```python
from build123d import *

# Parameters (mm, degrees)
F3_DEPTH = 32
F7_W     = 30
F7_H     = 8
F8_DEPTH = 4
F5_R     = 2.7
F9_DEPTH = 25


with BuildPart() as f1:
    # F0 (on Front) → F1 (revolve)
    with BuildSketch(Plane.XZ):
        Polygon((29.3, 16), (10.7, 16), (10.7, 13.35), (0, 13.35), (0, 0), (205, 0), (205, 12.5), (188.3, 12.5), (188.3, 12), (185.3, 12), (185.3, 14), (173.3, 14), (173.3, 13), (170.3, 13), (170.3, 14), (121.6, 14), (121.6, 13.3), (118.6, 13.3), (118.6, 16), (32.3, 16), (32.3, 15), (29.3, 15), align=None)
    revolve(axis=Axis((102.5, 0, 0), (-1, 0, 0)))

    # F2 (on face) → F3 (join)
    with BuildSketch(Plane(origin=(0, 0, 0), x_dir=(0, -1, 0), z_dir=(-1, 0, 0))):
        with BuildLine():
            ThreePointArc((-8.528071, 10.271052), (-6.675, 11.561439), (-4.630957, 12.521052))
            Line((-4.630957, 12.521052), (-5.630957, 14.253103))
            Line((-5.630957, 14.253103), (-9.146501, 16.842204))
            Line((-9.146501, 16.842204), (-10.012526, 16.342204))
            Line((-10.012526, 16.342204), (-9.528071, 12.003103))
            Line((-9.528071, 12.003103), (-8.528071, 10.271052))
        make_face()
        with BuildLine():
            Line((-2.25, 15.159027), (-2.25, 13.159027))
            ThreePointArc((-2.25, 13.159027), (0, 13.35), (2.25, 13.159027))
            Line((2.25, 13.159027), (2.25, 15.159027))
            Line((2.25, 15.159027), (0.5, 19.159027))
            Line((0.5, 19.159027), (-0.5, 19.159027))
            Line((-0.5, 19.159027), (-2.25, 15.159027))
        make_face()
        with BuildLine():
            Line((5.630957, 14.253103), (4.630957, 12.521052))
            ThreePointArc((4.630957, 12.521052), (6.675, 11.561439), (8.528071, 10.271052))
            Line((8.528071, 10.271052), (9.528071, 12.003103))
            Line((9.528071, 12.003103), (10.012526, 16.342204))
            Line((10.012526, 16.342204), (9.146501, 16.842204))
            Line((9.146501, 16.842204), (5.630957, 14.253103))
        make_face()
        with BuildLine():
            Line((12.003103, 9.528071), (10.271052, 8.528071))
            ThreePointArc((10.271052, 8.528071), (11.561439, 6.675), (12.521052, 4.630957))
            Line((12.521052, 4.630957), (14.253103, 5.630957))
            Line((14.253103, 5.630957), (16.842204, 9.146501))
            Line((16.842204, 9.146501), (16.342204, 10.012526))
            Line((16.342204, 10.012526), (12.003103, 9.528071))
        make_face()
        with BuildLine():
            Line((15.159027, 2.25), (13.159027, 2.25))
            ThreePointArc((13.159027, 2.25), (13.302171, 1.129045), (13.35, 0))
            ThreePointArc((13.35, 0), (13.302171, -1.129045), (13.159027, -2.25))
            Line((13.159027, -2.25), (15.159027, -2.25))
            Line((15.159027, -2.25), (19.159027, -0.5))
            Line((19.159027, -0.5), (19.159027, 0.5))
            Line((19.159027, 0.5), (15.159027, 2.25))
        make_face()
        with BuildLine():
            Line((14.253103, -5.630957), (12.521052, -4.630957))
            ThreePointArc((12.521052, -4.630957), (11.561439, -6.675), (10.271052, -8.528071))
            Line((10.271052, -8.528071), (12.003103, -9.528071))
            Line((12.003103, -9.528071), (16.342204, -10.012526))
            Line((16.342204, -10.012526), (16.842204, -9.146501))
            Line((16.842204, -9.146501), (14.253103, -5.630957))
        make_face()
        with BuildLine():
            Line((9.528071, -12.003103), (8.528071, -10.271052))
            ThreePointArc((8.528071, -10.271052), (6.675, -11.561439), (4.630957, -12.521052))
            Line((4.630957, -12.521052), (5.630957, -14.253103))
            Line((5.630957, -14.253103), (9.146501, -16.842204))
            Line((9.146501, -16.842204), (10.012526, -16.342204))
            Line((10.012526, -16.342204), (9.528071, -12.003103))
        make_face()
        with BuildLine():
            ThreePointArc((2.25, -13.159027), (0, -13.35), (-2.25, -13.159027))
            Line((-2.25, -13.159027), (-2.25, -15.159027))
            Line((-2.25, -15.159027), (-0.5, -19.159027))
            Line((-0.5, -19.159027), (0.5, -19.159027))
            Line((0.5, -19.159027), (2.25, -15.159027))
            Line((2.25, -15.159027), (2.25, -13.159027))
        make_face()
        with BuildLine():
            ThreePointArc((-4.630957, -12.521052), (-6.675, -11.561439), (-8.528071, -10.271052))
            Line((-8.528071, -10.271052), (-9.528071, -12.003103))
            Line((-9.528071, -12.003103), (-10.012526, -16.342204))
            Line((-10.012526, -16.342204), (-9.146501, -16.842204))
            Line((-9.146501, -16.842204), (-5.630957, -14.253103))
            Line((-5.630957, -14.253103), (-4.630957, -12.521052))
        make_face()
        with BuildLine():
            ThreePointArc((-10.271052, -8.528071), (-11.561439, -6.675), (-12.521052, -4.630957))
            Line((-12.521052, -4.630957), (-14.253103, -5.630957))
            Line((-14.253103, -5.630957), (-16.842204, -9.146501))
            Line((-16.842204, -9.146501), (-16.342204, -10.012526))
            Line((-16.342204, -10.012526), (-12.003103, -9.528071))
            Line((-12.003103, -9.528071), (-10.271052, -8.528071))
        make_face()
        with BuildLine():
            ThreePointArc((-13.159027, -2.25), (-13.35, 0), (-13.159027, 2.25))
            Line((-13.159027, 2.25), (-15.159027, 2.25))
            Line((-15.159027, 2.25), (-19.159027, 0.5))
            Line((-19.159027, 0.5), (-19.159027, -0.5))
            Line((-19.159027, -0.5), (-15.159027, -2.25))
            Line((-15.159027, -2.25), (-13.159027, -2.25))
        make_face()
        with BuildLine():
            ThreePointArc((-12.521052, 4.630957), (-11.561439, 6.675), (-10.271052, 8.528071))
            Line((-10.271052, 8.528071), (-12.003103, 9.528071))
            Line((-12.003103, 9.528071), (-16.342204, 10.012526))
            Line((-16.342204, 10.012526), (-16.842204, 9.146501))
            Line((-16.842204, 9.146501), (-14.253103, 5.630957))
            Line((-14.253103, 5.630957), (-12.521052, 4.630957))
        make_face()
        with BuildLine():
            ThreePointArc((2.25, 13.159027), (0, 13.35), (-2.25, 13.159027))
            ThreePointArc((-2.25, 13.159027), (-3.455234, 12.89511), (-4.630957, 12.521052))
            ThreePointArc((-4.630957, 12.521052), (-6.675, 11.561439), (-8.528071, 10.271052))
            ThreePointArc((-8.528071, 10.271052), (-9.439876, 9.439876), (-10.271052, 8.528071))
            ThreePointArc((-10.271052, 8.528071), (-11.561439, 6.675), (-12.521052, 4.630957))
            ThreePointArc((-12.521052, 4.630957), (-12.89511, 3.455234), (-13.159027, 2.25))
            ThreePointArc((-13.159027, 2.25), (-13.35, 0), (-13.159027, -2.25))
            ThreePointArc((-13.159027, -2.25), (-12.89511, -3.455234), (-12.521052, -4.630957))
            ThreePointArc((-12.521052, -4.630957), (-11.561439, -6.675), (-10.271052, -8.528071))
            ThreePointArc((-10.271052, -8.528071), (-9.439876, -9.439876), (-8.528071, -10.271052))
            ThreePointArc((-8.528071, -10.271052), (-6.675, -11.561439), (-4.630957, -12.521052))
            ThreePointArc((-4.630957, -12.521052), (-3.455234, -12.89511), (-2.25, -13.159027))
            ThreePointArc((-2.25, -13.159027), (0, -13.35), (2.25, -13.159027))
            ThreePointArc((2.25, -13.159027), (3.455234, -12.89511), (4.630957, -12.521052))
            ThreePointArc((4.630957, -12.521052), (6.675, -11.561439), (8.528071, -10.271052))
            ThreePointArc((8.528071, -10.271052), (9.439876, -9.439876), (10.271052, -8.528071))
            ThreePointArc((10.271052, -8.528071), (11.561439, -6.675), (12.521052, -4.630957))
            ThreePointArc((12.521052, -4.630957), (12.89511, -3.455234), (13.159027, -2.25))
            ThreePointArc((13.159027, -2.25), (13.302171, -1.129045), (13.35, 0))
            ThreePointArc((13.35, 0), (13.302171, 1.129045), (13.159027, 2.25))
            ThreePointArc((13.159027, 2.25), (12.89511, 3.455234), (12.521052, 4.630957))
            ThreePointArc((12.521052, 4.630957), (11.561439, 6.675), (10.271052, 8.528071))
            ThreePointArc((10.271052, 8.528071), (9.439876, 9.439876), (8.528071, 10.271052))
            ThreePointArc((8.528071, 10.271052), (6.675, 11.561439), (4.630957, 12.521052))
            ThreePointArc((4.630957, 12.521052), (3.455234, 12.89511), (2.25, 13.159027))
        make_face()
    extrude(amount=F3_DEPTH)

    # F7 (on offset) → F8 (cut)
    with BuildSketch(Plane.XZ.offset(14)):
        with Locations((135.3, 0)):
            Rectangle(F7_W, F7_H)
    extrude(amount=-F8_DEPTH, mode=Mode.SUBTRACT)

    # F5 (on offset) → F9 (cut)
    with BuildSketch(Plane.XZ.offset(12.5)):
        with Locations((193, 0)):
            Circle(F5_R)
    extrude(amount=-F9_DEPTH, mode=Mode.SUBTRACT)


solid = f1.part
```
Model file for the job. Use its own axes, mm. A direction names the side the tool comes from. Give positions to 0.01 mm unless a question says otherwise; leave off trailing zeros. Order: outer loops, then holes, each group sorted by start corner. A loop starts at its lowest first (then second) coordinate and runs counter-clockwise, first axis right, second up.
1) Saw through at A-A, the plane x = 193. Write the cut outline in (y, z).
2) 3-axis set-ups, long thin cutter, end or side, ignore diameter. For faces 4 (the flat face through (0, 8, -14)), 5 (the flat face through (0, 8, 14)), 6 (the cylindrical face through (120.079, 11.215, 7.15)), 7 (the flat face through (0, -8, 14)): which of +Z, -Z, +X, -X, +Y, -Y reach the whole face in a straight line?
3) Pin check, flat tips, straight feed: pin 1 (2 mm diameter, centred on x = -17, y = -14.5, fed in from +Z); pin 2 (5 mm diameter, centred on y = -16, z = 0, fed in from +X); pin 3 (1 mm diameter, centred on x = 97, z = -4.5, fed in from +Y). Stop position of each tip, or through.
4) Wall check: probe 1 along X at (y, z) = (0, 15.5); probe 2 along X at (y, z) = (-2, 0); probe 3 along X at (y, z) = (2, -13). Give the ranges that are in metal, low to high.
5) Mould opens along Z. For faces 1 (the flat face through (-15.78, 17.19, -1.36)), 2 (the flat face through (0, 14, -8)), 3 (the flat face through (-15.776, 14.142, 9.767)) say: +Z half, -Z half, draft (parallel to the pull), parting line (faces both ways), or undercut.
6) Saw through at B-B, the plane x = 90.5. Write the cut outline in (y, z).
Computed:
1. outline: (-12.2, -2.7) arc R12.5 ccw to (12.2, -2.7) - close; (-12.2, 2.7) - (12.2, 2.7) arc R12.5 ccw to start
2. face 4: -Z, +Y
2. face 5: +Z, +Y
2. face 6: none
2. face 7: +Z, -Y
3. pin 1: stops at z = 9.92
3. pin 2: stops at x = 185.3
3. pin 3: stops at y = 15.49
4. probe 1: x = -32 to 0, 10.7 to 29.3, 32.3 to 118.6
4. probe 2: x = -32 to 190.3, 195.7 to 205
4. probe 3: x = -32 to 170.3, 173.3 to 185.3
5. face 1: undercut
5. face 2: draft
5. face 3: +Z half
6. outline: circle Ø32 at (0, 0)
